```python
from build123d import *

# Parameters (mm, degrees)
SKETCH1_W             = 25.4
SKETCH1_H             = 25.4
SKETCH1_W_2           = 19.05
SKETCH1_H_2           = 19.05
BOSS_EXTRUDE1_DEPTH   = 203.2
CUT_EXTRUDE1_DEPTH    = 206.174779152
M10_CLEARANCE_HOLE1_D = 11


with BuildPart() as part:
    # Sketch1 → Boss-Extrude1 (new body)
    with BuildSketch(Plane.XY):
        Rectangle(SKETCH1_W, SKETCH1_H)
        Rectangle(SKETCH1_W_2, SKETCH1_H_2, mode=Mode.SUBTRACT)
    extrude(amount=BOSS_EXTRUDE1_DEPTH)

    # Sketch2 → Cut-Extrude1 (cut, through all)
    with BuildSketch(Plane(origin=(12.7, 0, 0), x_dir=(0, 0, -1), z_dir=(1, 0, 0))):
        Polygon((0, 12.7), (0, -12.7), (-25.4, 12.7), align=None)
    extrude(amount=-CUT_EXTRUDE1_DEPTH, mode=Mode.SUBTRACT)

    # M10 Clearance Hole1 (through all)
    with Locations(Plane(origin=(0, -12.7, 0), x_dir=(-1, 0, 0), z_dir=(0, -1, 0))):
        with Locations((0, -190.5)):
            Hole(M10_CLEARANCE_HOLE1_D / 2)


solid = part.part
```
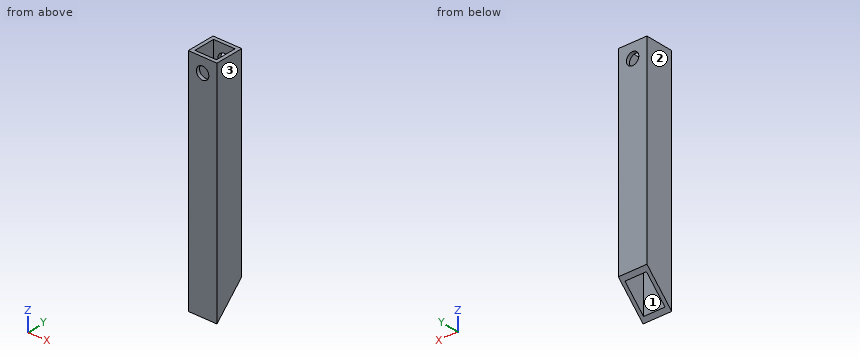
Geometry: final body of the model. Coordinates: model frame, mm. Face numbers are marked on the shaded views. Round coordinates to 2 decimals unless told otherwise and drop trailing zeros. Write each loop counter-clockwise with the first axis right and the second up, starting at its lowest first coordinate (ties: lowest second). Pieces come first, ordered by that corner, then holes.
Item 1: Section query C-C (y = -6). Return loops of the section in (x, z) (3 decimals), plus the area to 3 significant figures.
Item 2: Mould query, pull axis X, two halves, no side actions, for the marked faces 1, 2 and 3. Classes: +X half, -X half, draft (parallel to the pull), parting line (faces both ways), or undercut.
Item 3: Material intervals for L1, parallel to X at y = -6.75, z = 72 (3 decimals); L2, parallel to X at y = 11.2, z = 190.5, sorted ascending.
Item 4: Section query B-B (x = -7.5). Return loops of the section in (y, z) (3 decimals), plus the area to 3 significant figures.
Item 5: Section query D-D (z = 61.5). Return loops of the section in (x, y) (3 decimals).
Item 6: Pin query (flat end, axial travel): P1, Ø4, axis at x = 9, y = -8.5, coming from the +Z side. Return the tip coordinate at first contact, or that it passes through.
Item 7: Section query A-A (z = 190.5). Return loops of the section in (x, y) (3 decimals), plus the area to 3 significant figures.
Completed:
1. outline: (-12.7, 6.7) - (-9.525, 6.7) - (-9.525, 203.2) - (-12.7, 203.2) - close; (9.525, 6.7) - (12.7, 6.7) - (12.7, 203.2) - (9.525, 203.2) - close
1. area: 1,250 mm2
2. face 1: undercut
2. face 2: -X half
2. face 3: +X half
3. L1: x = -12.7 to -9.525, 9.525 to 12.7
3. L2: x = -12.7 to -5.5, 5.5 to 12.7
4. outline: (-12.7, 0) - (-9.525, 3.175) - (-9.525, 203.2) - (-12.7, 203.2) - close; (9.525, 22.225) - (12.7, 25.4) - (12.7, 203.2) - (9.525, 203.2) - close
4. area: 1,210 mm2
5. outline: (-12.7, -12.7) - (12.7, -12.7) - (12.7, 12.7) - (-12.7, 12.7) - close; hole (-9.525, -9.525) - (9.525, -9.525) - (9.525, 9.525) - (-9.525, 9.525) - close
6. P1: stops at z = 203.2
7. outline: (-12.7, -12.7) - (-5.5, -12.7) - (-5.5, -9.525) - (-9.525, -9.525) - (-9.525, 9.525) - (-5.5, 9.525) - (-5.5, 12.7) - (-12.7, 12.7) - close; (5.5, -12.7) - (12.7, -12.7) - (12.7, 12.7) - (5.5, 12.7) - (5.5, 9.525) - (9.525, 9.525) - (9.525, -9.525) - (5.5, -9.525) - close
7. area: 212 mm2
